Could you check a few things on this drawing? It's one solid part, dimensions in mm from its lowest x, y, z. Round coordinates to 2 decimals unless told otherwise and drop trailing zeros. Order: outer loops, then holes, each group sorted by start corner. A loop starts at its lowest first (then second) coordinate and runs counter-clockwise, first axis right, second up. Notation, with made-up numbers: (65.5, 38.25) -> (91.5, 38.25) arc R28 ccw to (91.5, 58.25) -> close; hole circle Ø8 at (17, 77). An arc over 180 degrees is marked (long way). Use a Markdown table: item, result. Add a question column.
(1) I'm going to push a flat-ended pin straight in: P1, Ø1, axis at x = 4, z = 2.5, coming from the +Y side. Where does the tip first touch, or does it pass through?
(2) If I drill on probe 1 along X at (y, z) = (0.3, 4); probe 2 along Z at (x, y) = (5, 0.7); probe 3 along X at (y, z) = (0.75, 4.75), over which ranges is the centre line in solid material (lowest first)?
(3) I want a section at A-A, the plane x = 7. Please give me the cut outline in (y, z), then the cut area to 3 significant figures.
(4) I want a section at B-B, the plane z = 4. Please give me the cut outline in (x, y).
(5) Thinking about a two-plate mould opening in Z: for the marked faces 1 and 2, which applies, pulls with the +Z half, pulls with the -Z half, needs draft (parallel to the pull), parting line crosses it, or undercut?
(6) I want a section at C-C, the plane y = 0.2. Please give me the cut outline in (x, z), then the cut area to 3 significant figures.
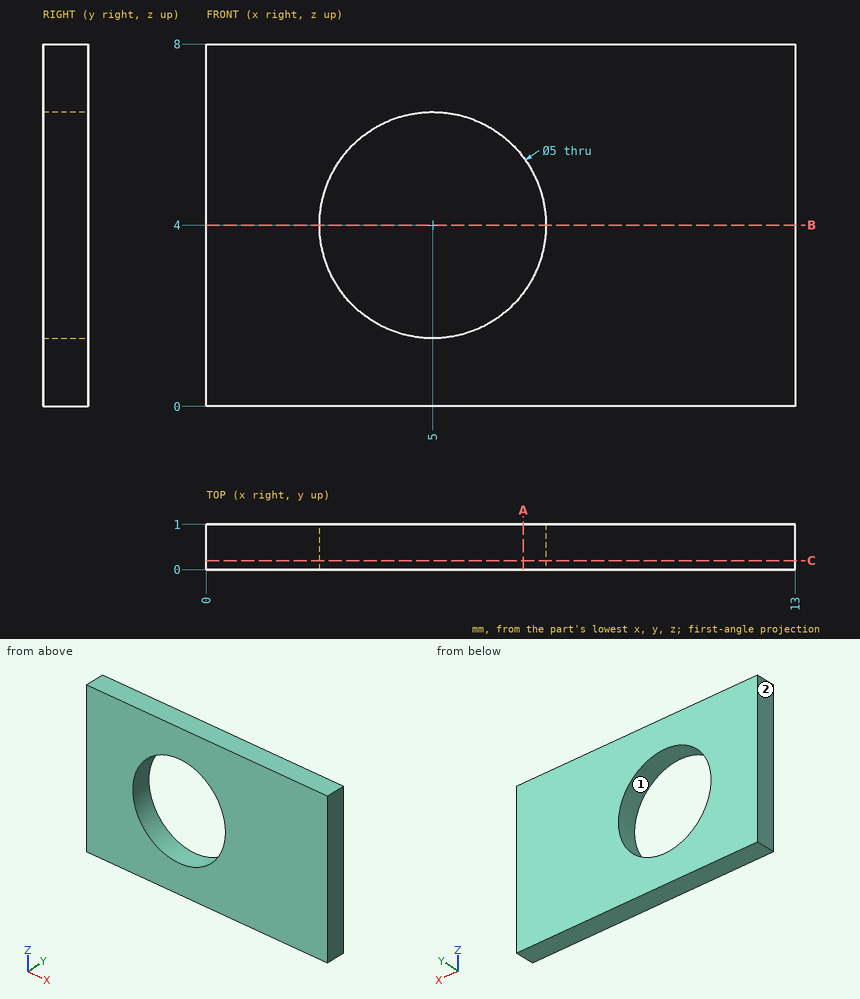
Taken from the geometry:
| question | item | result |
|---|---|---|
| 1 | P1 | passes through |
| 2 | probe 1 | x = 0 to 2.5, 7.5 to 13 |
| 2 | probe 2 | z = 0 to 1.5, 6.5 to 8 |
| 2 | probe 3 | x = 0 to 2.62, 7.38 to 13 |
| 3 | outline | (0, 0) -> (1, 0) -> (1, 2.5) -> (0, 2.5) -> close; (0, 5.5) -> (1, 5.5) -> (1, 8) -> (0, 8) -> close |
| 3 | area | 5.00 mm2 |
| 4 | outline | (0, 0) -> (2.5, 0) -> (2.5, 1) -> (0, 1) -> close; (7.5, 0) -> (13, 0) -> (13, 1) -> (7.5, 1) -> close |
| 5 | face 1 | undercut |
| 5 | face 2 | needs draft |
| 6 | outline | (0, 0) -> (13, 0) -> (13, 8) -> (0, 8) -> close; hole circle Ø5 at (5, 4) |
| 6 | area | 84.4 mm2 |
